Autodesk Inventor part; units mm, degrees
ref_plane "YZ Plane" through (0, 0, 0) normal (1, 0, 0) x (0, 1, 0)
ref_plane "XZ Plane" through (0, 0, 0) normal (0, 1, 0) x (-1, 0, 0)
ref_plane "XY Plane" through (0, 0, 0) normal (0, 0, 1) x (1, 0, 0)
sketch "Sketch1" plane through (0, 0, 0) normal (1, 0, 0) x (0, 1, 0)
  line L0 (0, 0) -> (38.1, 0)
  line L1 (38.1, 0) -> (38.1, -46.101)
  line L2 (38.1, -46.101) -> (0, -46.101)
  line L3 (0, -46.101) -> (0, 0)
  dimension "d0" = 38.1
  dimension "d1" = 46.101
extrude "Extrusion1" add sketch "Sketch1" along normal blind 3.175
sketch "Sketch2" plane through (3.175, 0, 0) normal (1, 0, 0) x (0, 0, -1)
  line L0 (0, 38.1) -> (0, 0) construction
  line L1 (0, 0) -> (46.101, 0) construction
  line L2 (46.101, 0) -> (46.101, 38.1) construction
  line L3 (46.101, 38.1) -> (0, 38.1) construction
  line L4 (0, 38.1) -> (0, 0) construction
  line L5 (0, 19.05) -> (46.101, 19.05) construction
  line L6 (46.101, 38.1) -> (0, 38.1) construction
  line L7 (0, 0) -> (46.101, 0) construction
  line L8 (46.101, 0) -> (46.101, 38.1)
  line L9 (23.0505, 19.05) -> (23.0505, 6.0641) construction
  line L10 (23.0505, 19.05) -> (23.0505, 32.0359) construction
  line L11 (17.0623, 6.0641) -> (23.0505, 6.0641) construction
  line L12 (23.0505, 6.0641) -> (29.0387, 6.0641) construction
  line L13 (17.0623, 6.0641) -> (17.0623, 7.2131) construction
  line L14 (29.0387, 6.0641) -> (29.0387, 7.2131) construction
  line L15 (29.0387, 6.0641) -> (35.0269, 6.0641) construction
  line L16 (35.0269, 6.0641) -> (41.0151, 6.0641) construction
  line L17 (41.0151, 6.0641) -> (41.0151, 7.2131) construction
  line L18 (17.0623, 6.0641) -> (11.0741, 6.0641) construction
  line L19 (11.0741, 6.0641) -> (5.0859, 6.0641) construction
  line L20 (5.0859, 7.2131) -> (5.0859, 6.0641) construction
  circle A0 centre (23.0505, 6.0641) radius 1.7859
  circle A1 centre (5.0859, 6.0641) radius 1.7859
  circle A2 centre (41.0151, 6.0641) radius 1.7859
  line L21 (5.0859, 6.0641) -> (5.0859, 32.0359) construction
  line L22 (5.0859, 32.0359) -> (23.0505, 32.0359) construction
  line L23 (23.0505, 32.0359) -> (41.0151, 32.0359) construction
  line L24 (41.0151, 32.0359) -> (41.0151, 6.0641) construction
  circle A3 centre (5.0859, 32.0359) radius 1.7859
  circle A4 centre (23.0505, 32.0359) radius 1.7859
  circle A5 centre (41.0151, 32.0359) radius 1.7859
  dimension "d16" = 3.5719
extrude "Extrusion2" cut sketch "Sketch2" against normal through all
sketch "Sketch3" plane through (3.175, 0, 0) normal (1, 0, 0) x (0, 0, -1)
  line L0 (0, 38.1) -> (0, 0)
  line L1 (0, 19.05) -> (46.101, 19.05)
  line L2 (46.101, 0) -> (46.101, 38.1)
  line L3 (0, 11.3401) -> (46.101, 11.3401)
  line L4 (46.101, 11.3401) -> (46.101, 26.7599)
  line L5 (46.101, 26.7599) -> (0, 26.7599)
  line L6 (0, 26.7599) -> (0, 11.3401)
  line L7 (0, 11.3401) -> (46.101, 26.7599) construction
  line L8 (46.101, 11.3401) -> (0, 26.7599) construction
  point P0 (23.0505, 19.05)
extrude "Extrusion3" add sketch "Sketch3" along normal blind 7.9375
sketch "Sketch4" plane through (0, 0, 0) normal (0, 0, 1) x (1, 0, 0)
  line L0 (0, 0) -> (0, 38.1)
  line L1 (0, 0) -> (3.175, 0)
  line L2 (3.175, 11.3401) -> (3.175, 0)
  line L3 (3.175, 11.3401) -> (11.1125, 11.3401)
  line L4 (11.1125, 26.7599) -> (11.1125, 11.3401)
  line L5 (3.175, 26.7599) -> (11.1125, 26.7599)
  line L6 (3.175, 38.1) -> (3.175, 26.7599)
  line L7 (0, 38.1) -> (3.175, 38.1)
  line L8 (3.175, 26.7599) -> (3.175, 11.3401)
  line L9 (11.1125, 19.05) -> (3.175, 19.05) construction
  line L10 (3.175, 26.7599) -> (11.1125, 26.7599) construction
  line L11 (7.1437, 26.7599) -> (7.1438, 11.3401) construction
  circle A0 centre (7.1438, 19.05) radius 2.3876
  dimension "d9" = 4.7752
extrude "Extrusion4" cut sketch "Sketch4" against normal through all contours A0
fillet "Fillet1" radius 3.175 2 edges at (11.1125, 26.7599, -23.0505) (11.1125, 11.3401, -23.0505)
fillet "Fillet2" radius 2.54 2 edges at (3.175, 26.7599, -23.0505) (3.175, 11.3401, -23.0505)
fillet "Fillet4" radius 5.715 4 edges at (1.5875, 0, -46.101) (1.5875, 0, 0) (1.5875, 38.1, 0) (1.5875, 38.1, -46.101)
properties part number "top axle holder 2"
Read the model definition and answer for the solid it produces. Units are mm, in the model's axes. A direction names the side the tool comes from. Coordinates: 2 decimals unless noted, no trailing zeros. Write each loop counter-clockwise with the first axis right and the second up, starting at its lowest first coordinate (ties: lowest second). Pieces come first, ordered by that corner, then holes. Notation, with made-up numbers: (24, -1) -> (62, -1) arc R35 ccw to (62, 32) -> close; hole circle Ø1 at (56, -27.75). An arc over 180 degrees is marked (long way). Return JSON: item names as keys, results as strings.
1. A cutting plane is placed at D-D (y = 33). Determine the outline of the cut face in (x, z) (3 decimals), and give its area (3 significant figures).
Found:
{"outline": "(0, -46.068) -> (3.175, -46.068) -> (3.175, -42.518) -> (0, -42.518) -> close; (0, -39.512) -> (3.175, -39.512) -> (3.175, -24.554) -> (0, -24.554) -> close; (0, -21.547) -> (3.175, -21.547) -> (3.175, -6.589) -> (0, -6.589) -> close; (0, -3.583) -> (3.175, -3.583) -> (3.175, -0.033) -> (0, -0.033) -> close", "area": "118 mm2"}
2. Find the intervals of material crossed by line 1 along X through (y, z) = (19, -13); line 2 along Z through (x, y) = (3, 32.5); line 3 along Y through (x, z) = (7, -6), in increasing order. Write a range as from..to.
Found:
{"line 1": "0..4.76, 9.53..11.11", "line 2": "-46.1..-42.74, -39.29..-24.78, -21.33..-6.81, -3.36..0", "line 3": "11.34..16.67, 21.43..26.76"}
3. A cutting plane is placed at A-A (y = 19.05). Determine the outline of the cut face in (x, z), and give its area (3 significant figures).
Found:
{"outline": "(0, -46.1) -> (4.76, -46.1) -> (4.76, 0) -> (0, 0) -> close; (9.53, -46.1) -> (11.11, -46.1) -> (11.11, 0) -> (9.53, 0) -> close", "area": "292 mm2"}
4. A cutting plane is placed at C-C (x = 9). Determine the outline of the cut face in (y, z), and give its area (3 significant figures).
Found:
{"outline": "(11.52, -46.1) -> (17.55, -46.1) -> (17.55, 0) -> (11.52, 0) -> close; (20.55, -46.1) -> (26.58, -46.1) -> (26.58, 0) -> (20.55, 0) -> close", "area": "556 mm2"}
5. A tool of negligible diameter and unlimited length cuts with its end or side. For faces 5 (the face through (7, 26.76, -23)), 6 (the face through (1.61, 36.47, -1.72)), 7 (the face through (3.175, 3, -23)), from which of +Z, -Z, +X, -X, +Y, -Y can it reach the whole face along a straight path? Write none if from no direction.
Found:
{"face 5": "+Z, -Z, +X, +Y", "face 6": "+Z, +X, -X, +Y", "face 7": "+Z, -Z, +X, -Y"}
6. Determine the mould class of faces 1 (the face through (1.61, 1.72, -1.63)), 2 (the face through (6.833, 21.417, -22.728)), 3 (the face through (10, 26, -23)), 4 (the face through (0, 19, -23)) for opening direction X: pulls with the +X half, pulls with the -X half, needs draft (parallel to the pull), parting line crosses it, or undercut.
Found:
{"face 1": "needs draft", "face 2": "undercut", "face 3": "pulls with the +X half", "face 4": "pulls with the -X half"}
7. Each of these flat-tipped pins is pushed along its axis until it touches: P1, Ø0.7, axis at x = 7, z = -32.5, coming from the -Y side; P2, Ø3, axis at y = 32.04, z = -41.02, coming from the +X side; P3, Ø4.5, axis at y = 6, z = -23.5, coming from the +X side (3 decimals); P4, Ø0.7, axis at x = 6.5, z = -21.5, coming from the +Y side. Where does it stop, or does it pass through?
Found:
{"P1": "y = 11.34", "P2": "through", "P3": "x = 3.175", "P4": "y = 26.76"}
